Could you check a few things on this model? Use its own coordinates, in mm. A direction names the side the tool comes from. Coordinates: 2 decimals unless noted, no trailing zeros. Loops run counter-clockwise (first coordinate to the right, second up) from the corner with the lowest first, then second, coordinate; pieces in that order, holes last. Notation, with made-up numbers: M -12.5,81 L 2.5,81 A26 cw 2.5,100 Z; hole C -13.5,46.5 d9. An arc over 180 degrees is marked long. Use one line per item in the form item = value. Start each with the question number.
```python
from build123d import *

# Parameters (mm, degrees)
SKETCH1_W           = 22
SKETCH1_H           = 17.1
BOSS_EXTRUDE1_DEPTH = 12.05
CUT_EXTRUDE1_START  = 8.55
SKETCH2_R           = 2.77735613
SKETCH2_W           = 4.746499011
SKETCH2_H           = 3.149119536
SKETCH2_W_2         = 4.518301943
CUT_EXTRUDE1_DEPTH  = 1


with BuildPart() as part:
    # Sketch1 → Boss-Extrude1 (new body)
    with BuildSketch(Plane.XY):
        Rectangle(SKETCH1_W, SKETCH1_H)
    extrude(amount=BOSS_EXTRUDE1_DEPTH)

    # Sketch2 → Cut-Extrude1 (cut)
    with BuildSketch(Plane(origin=(0, 0, 0), x_dir=(1, 0, 0), z_dir=(0, 1, 0)).offset(CUT_EXTRUDE1_START)):
        with Locations(Location((0, -6, 0), (0, 0, 90))):
            Circle(SKETCH2_R)
        with Locations((6.663354381, -6)):
            Rectangle(SKETCH2_W, SKETCH2_H)
        with Locations((-6.663354381, -6)):
            Rectangle(SKETCH2_W_2, SKETCH2_H)
    extrude(amount=-CUT_EXTRUDE1_DEPTH, mode=Mode.SUBTRACT)


solid = part.part
```
Item 1: Thinking about a two-plate mould opening in X: for faces 1 (the flat face through (11, 0, 6)), 2 (the flat face through (9.037, 8, 6)), 3 (the flat face through (-7, 8, 4.425)), 4 (the flat face through (-3, 8.55, 5)), which applies, pulls with the +X half, pulls with the -X half, needs draft (parallel to the pull), parting line crosses it, or undercut?
Item 2: For faces 5 (the cylindrical face through (-2.342, 8.057, 4.507)), 6 (the flat face through (0, 0, 12.05)), which set-ups out of +Z, -Z, +X, -X, +Y, -Y let a thin tool reach every point of the face, with its end or its side?
Item 3: Please list where these lines run through material, in increasing order: line 1 along X through (y, z) = (7.9, 6); line 2 along Y through (x, z) = (9, 5.75).
Item 4: I want a section at C-C (x = -0.5). Write out the boundary of the cut face in (y, z).
Item 5: I want a section at A-A (x = 7.5). Write out the boundary of the cut face in (y, z), plus the area to 3 significant figures.
Item 6: I'm going to push a flat-ended pin straight in: P1, Ø3, axis at x = -1, z = 5.5, coming from the +Y side. Where does the tip first touch, or does it pass through?
Item 7: I want a section at B-B (z = 6). Write out the boundary of the cut face in (x, y).
Worked answers:
q1.face_1 = pulls with the +X half
q1.face_2 = undercut
q1.face_3 = undercut
q1.face_4 = needs draft
q2.face_5 = +Y
q2.face_6 = +Z, +X, -X, +Y, -Y
q3.line_1 = -11 to -8.92, -4.4 to -2.78, 2.78 to 4.29, 9.04 to 11
q3.line_2 = -8.55 to 7.55
q4.outline = M -8.55,0 L 8.55,0 L 8.55,3.27 L 7.55,3.27 L 7.55,8.73 L 8.55,8.73 L 8.55,12.05 L -8.55,12.05 Z
q5.outline = M -8.55,0 L 8.55,0 L 8.55,4.43 L 7.55,4.43 L 7.55,7.57 L 8.55,7.57 L 8.55,12.05 L -8.55,12.05 Z
q5.area = 203 mm²
q6.P1 = 7.55
q7.outline = M -11,-8.55 L 11,-8.55 L 11,8.55 L 9.04,8.55 L 9.04,7.55 L 4.29,7.55 L 4.29,8.55 L 2.78,8.55 L 2.78,7.55 L -2.78,7.55 L -2.78,8.55 L -4.4,8.55 L -4.4,7.55 L -8.92,7.55 L -8.92,8.55 L -11,8.55 Z
